```python
from build123d import *

# Parameters (mm, degrees)
SKETCH2_W           = 53.86
SKETCH2_H           = 95.04
BOSS_EXTRUDE1_DEPTH = 3
SKETCH3_W           = 70
SKETCH3_H           = 110
SKETCH3_R           = 1.25
BOSS_EXTRUDE2_DEPTH = 1


with BuildPart() as part:
    # Sketch2 → Boss-Extrude1 (new body)
    with BuildSketch(Plane.XY):
        with Locations((6.912993197, -3.934965986)):
            Rectangle(SKETCH2_W, SKETCH2_H)
    extrude(amount=BOSS_EXTRUDE1_DEPTH)

    # Sketch3 → Boss-Extrude2 (add)
    with BuildSketch(Plane(origin=(0, 0, 0), x_dir=(-1, 0, 0), z_dir=(0, 0, -1))):
        with Locations((-6.912993197, -3.934965986)):
            Rectangle(SKETCH3_W, SKETCH3_H)
        with Locations((24.922942909, 46.09293361)):
            Circle(SKETCH3_R, mode=Mode.SUBTRACT)
        with Locations((24.922942909, -53.962865582)):
            Circle(SKETCH3_R, mode=Mode.SUBTRACT)
        with Locations(Location((-38.748929304, 46.09293361, 0), (0, 0, 180))):
            Circle(SKETCH3_R, mode=Mode.SUBTRACT)
        with Locations(Location((-38.748929304, -53.962865582, 0), (0, 0, 180))):
            Circle(SKETCH3_R, mode=Mode.SUBTRACT)
    extrude(amount=BOSS_EXTRUDE2_DEPTH)


solid = part.part
```
The model under review builds one solid part; all positions refer to its coordinate system, in mm. A direction names the side the tool comes from. Round coordinates to 2 decimals unless told otherwise and drop trailing zeros. Loops run counter-clockwise (first coordinate to the right, second up) from the corner with the lowest first, then second, coordinate; pieces in that order, holes last. Notation, with made-up numbers: M 20,73.5 L 48,73.5 A24 ccw 48,103.5 Z; hole C 24,10.25 d9. An arc over 180 degrees is marked long. Answer as a JSON object with one key per item and string values.
(1) Clearance check with flat-ended pins moving along their axes: P1, Ø3, axis at x = 38.75, y = -53.96, coming from the -Z side; P2, Ø3, axis at x = -24.92, y = -53.96, coming from the +Z side; P3, Ø1.5, axis at x = 15.5, z = 1, coming from the -Y side; P4, Ø0.9, axis at y = -9.5, z = 1.5, coming from the -X side. State where each tip first meets the part, or that it passes through.
Resolved:
{"P1": "z = -1", "P2": "z = 0", "P3": "y = -51.45", "P4": "x = -20.02"}
(2) Take a section at A-A on x = 14. Give the boundary of the cut face in (y, z).
Resolved:
{"outline": "M -58.93,-1 L 51.07,-1 L 51.07,0 L 43.59,0 L 43.59,3 L -51.45,3 L -51.45,0 L -58.93,0 Z"}
(3) To check wall thickness, follow line 1 along X through (y, z) = (-54, -0.4); line 2 along Y through (x, z) = (8, 0.8); line 3 along X through (y, z) = (-50, 2.4). State the ranges of each line that lie inside material, in increasing order.
Resolved:
{"line 1": "-28.09 to -26.17, -23.67 to 37.5, 40 to 41.91", "line 2": "-51.45 to 43.59", "line 3": "-20.02 to 33.84"}
(4) Draft analysis for pull direction X (two halves, no side actions). For faces 1 (the cylindrical face through (38.586, -55.202, -0.493)), 2 (the flat face through (7, 43.585, 1)), 3 (the flat face through (33.843, -5, 1)), state which applies: released by +X, released by -X, zero draft, split by the parting line, or undercut.
Resolved:
{"face 1": "undercut", "face 2": "zero draft", "face 3": "released by +X"}
(5) Take a section at C-C on z = 0.75. Give the boundary of the cut face in (x, y).
Resolved:
{"outline": "M -20.02,-51.45 L 33.84,-51.45 L 33.84,43.59 L -20.02,43.59 Z"}
(6) Take a section at B-B on y = 17.5. Give the boundary of the cut face in (x, z), and give its area (3 significant figures).
Resolved:
{"outline": "M -28.09,-1 L 41.91,-1 L 41.91,0 L 33.84,0 L 33.84,3 L -20.02,3 L -20.02,0 L -28.09,0 Z", "area": "232 mm²"}
(7) Tool access review of faces 4 (the flat face through (7, -51.455, 1)), 5 (the cylindrical face through (-25.5, 44.984, -0.493)), 6 (the flat face through (-20.017, -5, 1)): name each direction out of +Z, -Z, +X, -X, +Y, -Y from which nothing blocks a thin tool from reaching the whole face with its end or side.
Resolved:
{"face 4": "+Z, +X, -X, -Y", "face 5": "+Z, -Z", "face 6": "+Z, -X, +Y, -Y"}
